For this review, take the finished solid that the model builds, in its own axes (mm). A direction names the side the tool comes from. Give positions to 0.01 mm unless a question says otherwise; leave off trailing zeros. Write each loop counter-clockwise with the first axis right and the second up, starting at its lowest first coordinate (ties: lowest second). Pieces come first, ordered by that corner, then holes.
Autodesk Inventor part; units mm, degrees
ref_plane "YZ Plane" through (0, 0, 0) normal (1, 0, 0) x (0, 1, 0)
ref_plane "XZ Plane" through (0, 0, 0) normal (0, 1, 0) x (-1, 0, 0)
ref_plane "XY Plane" through (0, 0, 0) normal (0, 0, 1) x (1, 0, 0)
sketch "Boceto principal" plane through (0, 0, 0) normal (1, 0, 0) x (0, 1, 0)
  line L0 (0, 0) -> (0, -1)
  line L1 (0, -1) -> (3.5, -1)
  line L2 (4, -1.5) -> (4, -7)
  line L3 (4.5, -7.5) -> (30.5, -7.5)
  line L4 (31, -7) -> (31, -1.5)
  line L5 (31.5, -1) -> (35, -1)
  line L6 (35, -1) -> (35, 0)
  line L7 (35, 0) -> (30.5, 0)
  line L8 (30, -0.5) -> (30, -6)
  line L9 (29.5, -6.5) -> (5.5, -6.5)
  line L10 (5, -6) -> (5, -0.5)
  line L11 (4.5, 0) -> (0, 0)
  arc A0 (4, -1.5) -> (3.5, -1) centre (3.5, -1.5) ccw
  arc A1 (4, -7) -> (4.5, -7.5) centre (4.5, -7) ccw
  arc A2 (30.5, -7.5) -> (31, -7) centre (30.5, -7) ccw
  arc A3 (31.5, -1) -> (31, -1.5) centre (31.5, -1.5) ccw
  arc A4 (30.5, 0) -> (30, -0.5) centre (30.5, -0.5) ccw
  arc A5 (29.5, -6.5) -> (30, -6) centre (29.5, -6) ccw
  arc A6 (5, -6) -> (5.5, -6.5) centre (5.5, -6) ccw
  arc A7 (5, -0.5) -> (4.5, 0) centre (4.5, -0.5) ccw
extrude "Extrusion1" add sketch "Boceto principal" along normal blind 184.25
sketch "Boceto agujeros" plane through (0, 0, 0) normal (0, 0, 1) x (1, 0, 0)
  line L0 (7.6, 14.9) -> (20.4, 14.9)
  line L1 (20.4, 20.1) -> (7.6, 20.1)
  arc A0 (7.6, 20.1) -> (7.6, 14.9) centre (7.6, 17.5) ccw
  arc A1 (20.4, 14.9) -> (20.4, 20.1) centre (20.4, 17.5) ccw
extrude "Extrusion2" cut sketch "Boceto agujeros" against normal blind 15
pattern_linear "Rectangular Pattern1" count 8 spacing 25 along (1, 0, 0) of "Extrusion2"
properties part number "Riel120mm"
(1) We need section C-C (y = 17.5). Count the separate pieces of the cut face and the enclosed holes in it, and give its area (3 significant figures).
(2) We need section A-A (z = -4). Write out the cut boundary in (x, y).
(3) Clearance check with flat-ended pins moving along their axes: pin 1 Ø0.8 at (x, z) = (40.5, -7) entering from -Y; pin 2 Ø3 at (x, y) = (47.5, 2) entering from -Z; pin 3 Ø0.8 at (x, z) = (138, -7) entering from +Y. State where each tip first meets the part, or that it passes through.
(4) The part is to be moulded in two halves that separate along Y. For faces 6 (the flat face through (91, 5, -3)), 7 (the flat face through (90.8, 20.3, -6.5)), 8 (the flat face through (184.25, 29, -7)), 9 (the flat face through (91, 4, -4)), say which applies: +Y half, -Y half, draft (parallel to the pull), parting line (faces both ways), or undercut.
(5) Tool access review of faces 1 (the flat face through (91, 2, 0)), 2 (the flat face through (0, 17, -7)), 3 (the flat face through (91, 2, -1)), 4 (the flat face through (91, 33, -1)), 5 (the flat face through (91, 30, -3)): name each direction out of +Z, -Z, +X, -X, +Y, -Y from which nothing blocks a thin tool from reaching the whole face with its end or side.
(6) For L1, parallel to Y at x = 120.5, z = -7; L2, parallel to Y at x = 76.5, z = -2; L3, parallel to Z at x = 117, y = 12.5, list the stretches that pass through material, from the lowest coordinate up.
(7) We need section B-B (x = 110.5). Write out the cut boundary in (y, z).
The answers:
1. separate pieces: 8
1. enclosed holes: 0
1. area: 54.0 mm2
2. outline: (0, 4) - (184.25, 4) - (184.25, 5) - (0, 5) - close; (0, 30) - (184.25, 30) - (184.25, 31) - (0, 31) - close
3. pin 1: stops at y = 4
3. pin 2: stops at z = -1
3. pin 3: stops at y = 31
4. face 6: undercut
4. face 7: undercut
4. face 8: draft
4. face 9: -Y half
5. face 1: +Z, +X, -X, +Y, -Y
5. face 2: +Z, -Z, -X, +Y, -Y
5. face 3: -Z, +X, -X, -Y
5. face 4: -Z, +X, -X, +Y
5. face 5: +Z, +X, -X
6. L1: y = 4 to 14.9, 20.1 to 31
6. L2: y = 4 to 5, 30 to 31
6. L3: z = -7.5 to -6.5
7. outline: (0, -1) - (3.5, -1) arc R0.5 cw to (4, -1.5) - (4, -7) arc R0.5 ccw to (4.5, -7.5) - (14.9, -7.5) - (14.9, -6.5) - (5.5, -6.5) arc R0.5 cw to (5, -6) - (5, -0.5) arc R0.5 ccw to (4.5, 0) - (0, 0) - close; (20.1, -7.5) - (30.5, -7.5) arc R0.5 ccw to (31, -7) - (31, -1.5) arc R0.5 cw to (31.5, -1) - (35, -1) - (35, 0) - (30.5, 0) arc R0.5 ccw to (30, -0.5) - (30, -6) arc R0.5 cw to (29.5, -6.5) - (20.1, -6.5) - close
